The listing builds one solid part. Answer for the finished solid, in the listing's coordinates (mm). A direction names the side the tool comes from. Coordinates: 2 decimals unless noted, no trailing zeros. Order: outer loops, then holes, each group sorted by start corner. A loop starts at its lowest first (then second) coordinate and runs counter-clockwise, first axis right, second up.
from build123d import *

# Parameters (mm, degrees)
SKETCH1_R           = 3.5
BOSS_EXTRUDE2_DEPTH = 4


with BuildPart() as part:
    # Sketch1 → Boss-Extrude2 (new body)
    with BuildSketch(Plane.XY):
        with BuildLine():
            Line((0, 7.5), (-9.088423691, 4))
            Line((-9.088423691, 4), (-42.311576309, 4))
            Line((-42.311576309, 4), (-51.4, 7.5))
            ThreePointArc((-51.4, 7.5), (-58.9, 0), (-51.4, -7.5))
            Line((-51.4, -7.5), (-42.311576309, -4))
            Line((-42.311576309, -4), (-9.088423691, -4))
            Line((-9.088423691, -4), (0, -7.5))
            ThreePointArc((0, -7.5), (7.5, 0), (0, 7.5))
        make_face()
        Circle(SKETCH1_R, mode=Mode.SUBTRACT)
        with Locations((-51.4, 0)):
            Circle(SKETCH1_R, mode=Mode.SUBTRACT)
    extrude(amount=BOSS_EXTRUDE2_DEPTH)


solid = part.part
1) Each of these flat-tipped pins is pushed along its axis until it touches: P1, Ø2, axis at x = -19.5, z = 2.5, coming from the -Y side; P2, Ø2, axis at y = 5.5, z = 1.5, coming from the +X side; P3, Ø1, axis at y = 3.5, z = 3, coming from the -X side. Where does it stop, or does it pass through?
2) Section D-D (y = -1) is taken. Give the vertices of the cut face in (x, z).
3) Section A-A (z = 1) is taken. Give the vertices of the cut face in (x, y), then the cut area to 3 significant figures.
4) Section B-B (y = -6) is taken. Give the vertices of the cut face in (x, z), then the cut area to 3 significant figures.
5) Determine the mould class of faces 1 (the face through (-4.481, 5.774, 1.972)), 2 (the face through (-48.06, 1.05, 1.97)), 3 (the face through (-4.608, -5.726, 1.972)) for opening direction Y: released by +Y, released by -Y, zero draft, split by the parting line, or undercut.
6) Consider L1, parallel to Y at x = -51.4, z = 2.25; L2, parallel to X at y = 2, z = 2.65; L3, parallel to Y at x = -37, z = 3.6. Determine where each line is inside the solid, lowest interval first.
7) Section C-C (x = -50) is taken. Give the vertices of the cut face in (y, z), then the cut area to 3 significant figures.
8) A tool of negligible diameter and unlimited length cuts with its end or side. For faces 4 (the face through (-25, 4, 2)), 5 (the face through (-26, -4, 2)), 6 (the face through (7.5, -0.16, 1.97)), from which of +Z, -Z, +X, -X, +Y, -Y can it reach the whole face along a straight path? Write none if from no direction.
Filled sheet:
1. P1: stops at y = -4
1. P2: stops at x = 6
1. P3: stops at x = -58.27
2. outline: (-58.83, 0) - (-54.75, 0) - (-54.75, 4) - (-58.83, 4) - close; (-48.05, 0) - (-3.35, 0) - (-3.35, 4) - (-48.05, 4) - close; (3.35, 0) - (7.43, 0) - (7.43, 4) - (3.35, 4) - close
3. outline: (-51.4, -7.5) - (-42.31, -4) - (-9.09, -4) - (0, -7.5) arc R7.5 ccw to (0, 7.5) - (-9.09, 4) - (-42.31, 4) - (-51.4, 7.5) arc R7.5 ccw to start; hole circle Ø7 at (-51.4, 0); hole circle Ø7 at (0, 0)
3. area: 575 mm2
4. outline: (-55.9, 0) - (-47.5, 0) - (-47.5, 4) - (-55.9, 4) - close; (-3.9, 0) - (4.5, 0) - (4.5, 4) - (-3.9, 4) - close
4. area: 67.2 mm2
5. face 1: released by +Y
5. face 2: undercut
5. face 3: released by -Y
6. L1: y = -7.5 to -3.5, 3.5 to 7.5
6. L2: x = -58.63 to -54.27, -48.53 to -2.87, 2.87 to 7.23
6. L3: y = -4 to 4
7. outline: (-6.96, 0) - (-3.21, 0) - (-3.21, 4) - (-6.96, 4) - close; (3.21, 0) - (6.96, 0) - (6.96, 4) - (3.21, 4) - close
7. area: 30.0 mm2
8. face 4: +Z, -Z, +Y
8. face 5: +Z, -Z, -Y
8. face 6: +Z, -Z, +X
